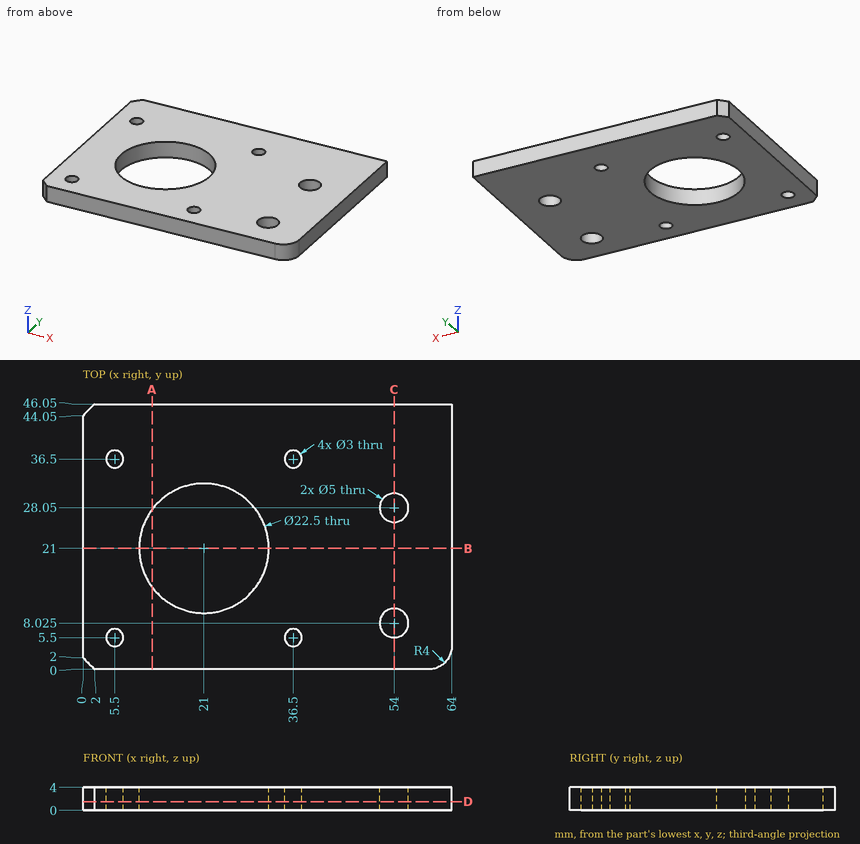
Source: three-view drawing plus pictorial views. Frame: mm from the lowest corner of the part. Round coordinates to 2 decimals unless told otherwise and drop trailing zeros. Loops run counter-clockwise (first coordinate to the right, second up) from the corner with the lowest first, then second, coordinate; pieces in that order, holes last. Notation, with made-up numbers: (88, 44) - (119, 44) arc R10 ccw to (119, 61) - close; hole circle Ø2 at (67.5, 82.5). An arc over 180 degrees is marked (long way). Write each question's results on one line, items separated by ' | '. Start each with the question number.
1) Line query: probe 1 along X at (y, z) = (28.05, 0.95); probe 2 along X at (y, z) = (37, 1.55); probe 3 along X at (y, z) = (8, 0.4). Output: solid intervals per line, ascending. Write a range as [from, to].
2) Cut plane C-C on x = 54. Return loops of the section in (y, z) (3 decimals).
3) Cut plane A-A on x = 12. Return loops of the section in (y, z), then the cut area to 3 significant figures.
4) Cut plane D-D on z = 1.5. Return loops of the section in (x, y) (3 decimals).
5) Cut plane B-B on y = 21. Return loops of the section in (x, z).
Verdict:
1) probe 1: x = [0, 12.23], [29.77, 51.5], [56.5, 64] | probe 2: x = [0, 4.09], [6.91, 35.09], [37.91, 64] | probe 3: x = [0, 51.5], [56.5, 64]
2) outline: (0, 0) - (5.525, 0) - (5.525, 4) - (0, 4) - close; (10.525, 0) - (25.55, 0) - (25.55, 4) - (10.525, 4) - close; (30.55, 0) - (46.05, 0) - (46.05, 4) - (30.55, 4) - close
3) outline: (0, 0) - (14.25, 0) - (14.25, 4) - (0, 4) - close; (27.75, 0) - (46.05, 0) - (46.05, 4) - (27.75, 4) - close | area: 130 mm2
4) outline: (0, 2) - (2, 0) - (60, 0) arc R4 ccw to (64, 4) - (64, 46.05) - (2, 46.05) - (0, 44.05) - close; hole circle Ø3 at (5.5, 5.5); hole circle Ø3 at (5.5, 36.5); hole circle Ø22.5 at (21, 21); hole circle Ø3 at (36.5, 5.5); hole circle Ø3 at (36.5, 36.5); hole circle Ø5 at (54, 8.025); hole circle Ø5 at (54, 28.05)
5) outline: (0, 0) - (9.75, 0) - (9.75, 4) - (0, 4) - close; (32.25, 0) - (64, 0) - (64, 4) - (32.25, 4) - close
